Can you work these out from the model? Positions are in its coordinate system, mm. A direction names the side the tool comes from. Round coordinates to 2 decimals unless told otherwise and drop trailing zeros. Write each loop counter-clockwise with the first axis right and the second up, starting at its lowest first coordinate (ties: lowest second). Pieces come first, ordered by that corner, then holes. Notation, with made-up numbers: M 40.5,76.5 L 88.5,76.5 A13 ccw 88.5,83.5 Z; hole C 29.25,40.25 d11. An arc over 180 degrees is marked long. Answer as a JSON object with one key per item and string values. Group by question number.
1) On a 3-axis mill with a long thin cutter (end or side, diameter ignored), from which of +Z, -Z, +X, -X, +Y, -Y can I reach the whole of each face in a straight line? I mean faces 4 (the flat face through (-216.344, -6, 2)), 5 (the flat face through (-97.68, -44, 2)), 6 (the flat face through (-161, -142.256, 2)). Say none if no direction works.
2) Suppose I cut it at A-A, the plane y = -97. Write out the boundary of the cut face in (x, z), and give its area (3 significant figures).
3) Suppose I cut it at B-B, the plane z = 2.7. State how many separate pieces and enclosed holes the cut face has, and give its area (3 significant figures).
4) Suppose I cut it at C-C, the plane y = -68. Write out the boundary of the cut face in (x, z), and give its area (3 significant figures).
5) Please list where these lines run through material, in increasing order: L1, parallel to X at y = -116.5, z = 1.4; L2, parallel to Y at x = -112, z = 1.4; L3, parallel to X at y = -23.5, z = 1.8. Write a range as [from, to].
6) If we mould it in two halves opening along X, with no side actions, what happens to faces 1 (the flat face through (-100.68, -9, 2)), 2 (the flat face through (-116, -1.256, 2)), 3 (the flat face through (-87.68, -73, 2))? For each: +X half, -X half, draft (parallel to the pull), parting line (faces both ways), or undercut.
7) Suppose I cut it at D-D, the plane x = -163. Write out the boundary of the cut face in (y, z).
from build123d import *

# Parameters (mm, degrees)
F0_W     = 3
F0_H     = 5
F1_DEPTH = 4


with BuildPart() as f1:
    # F0 (on Top) → F1 (new body)
    with BuildSketch(Plane.XY):
        with BuildLine():
            Line((-228.3440142274, -137.3912245035), (-231.3440142274, -137.3912245035))
            Line((-231.3440142274, -137.3912245035), (-231.3440142274, -142.256315279))
            Line((-231.3440142274, -142.256315279), (-226.3440142274, -142.256315279))
            Line((-226.3440142274, -142.256315279), (-226.3440142274, -139.3912245035))
            ThreePointArc((-226.3440142274, -139.3912245035), (-227.7582277898, -138.8054380659), (-228.3440142274, -137.3912245035))
        make_face()
        with BuildLine():
            Line((-87.6802765131, -142.256315279), (-87.6802765131, -137.256315279))
            Line((-87.6802765131, -137.256315279), (-90.6802765131, -137.256315279))
            ThreePointArc((-90.6802765131, -137.256315279), (-91.2660629507, -138.6705288414), (-92.6802765131, -139.256315279))
            Line((-92.6802765131, -139.256315279), (-92.6802765131, -142.256315279))
            Line((-92.6802765131, -142.256315279), (-87.6802765131, -142.256315279))
        make_face()
        with BuildLine():
            Line((-87.6802765131, -1.256315279), (-92.6802765131, -1.256315279))
            Line((-92.6802765131, -1.256315279), (-92.6802765131, -4.256315279))
            ThreePointArc((-92.6802765131, -4.256315279), (-91.2660629507, -4.8421017166), (-90.6802765131, -6.256315279))
            Line((-90.6802765131, -6.256315279), (-87.6802765131, -6.256315279))
            Line((-87.6802765131, -6.256315279), (-87.6802765131, -1.256315279))
        make_face()
        with BuildLine():
            Line((-134.6802765131, -1.256315279), (-139.6802765131, -1.256315279))
            Line((-139.6802765131, -1.256315279), (-139.6802765131, -6.256315279))
            Line((-139.6802765131, -6.256315279), (-136.6802765131, -6.256315279))
            ThreePointArc((-136.6802765131, -6.256315279), (-136.0944900755, -4.8421017166), (-134.6802765131, -4.256315279))
            Line((-134.6802765131, -4.256315279), (-134.6802765131, -1.256315279))
        make_face()
        with BuildLine():
            Line((-221.3440142274, -132.256315279), (-231.3440142274, -132.256315279))
            Line((-231.3440142274, -132.256315279), (-231.3440142274, -137.3912245035))
            Line((-231.3440142274, -137.3912245035), (-228.3440142274, -137.3912245035))
            ThreePointArc((-228.3440142274, -137.3912245035), (-226.3440142274, -135.3912245035), (-224.3440142274, -137.3912245035))
            ThreePointArc((-224.3440142274, -137.3912245035), (-224.929800665, -138.8054380659), (-226.3440142274, -139.3912245035))
            Line((-226.3440142274, -139.3912245035), (-226.3440142274, -142.256315279))
            Line((-226.3440142274, -142.256315279), (-221.3440142274, -142.256315279))
            Line((-221.3440142274, -142.256315279), (-221.3440142274, -132.256315279))
        make_face()
        Polygon((-217.9440142274, -132.256315279), (-221.3440142274, -132.256315279), (-221.3440142274, -142.256315279), (-139.3440142274, -142.256315279), (-139.4949736476, -132.256315279), (-142.7440142274, -132.256315279), (-147.4240142274, -132.256315279), (-151.4240142274, -132.256315279), align=None)
        Polygon((-216.3440142274, -11.256315279), (-216.3440142274, -1.256315279), (-221.3440142274, -1.256315279), (-221.3440142274, -6.256315279), (-221.3440142274, -11.256315279), (-217.9440142274, -11.256315279), align=None)
        Polygon((-139.6802765131, -6.256315279), (-139.6802765131, -1.256315279), (-144.6802765131, -1.256315279), (-144.6802765131, -11.256315279), (-142.7440142274, -11.256315279), (-139.6802765131, -11.256315279), align=None)
        Polygon((-134.3440142274, -124.756315279), (-139.3440142274, -124.756315279), (-139.3440142274, -128.856315279), (-139.3440142274, -132.256315279), (-139.4949736476, -132.256315279), (-139.3440142274, -142.256315279), (-129.6802765131, -142.256315279), (-129.6802765131, -124.756315279), align=None)
        with BuildLine():
            Line((-221.3440142274, -6.256315279), (-221.3440142274, -1.256315279))
            Line((-221.3440142274, -1.256315279), (-231.3440142274, -1.256315279))
            Line((-231.3440142274, -1.256315279), (-231.3440142274, -132.256315279))
            Line((-231.3440142274, -132.256315279), (-221.3440142274, -132.256315279))
            Line((-221.3440142274, -132.256315279), (-221.3440142274, -128.856315279))
            Line((-221.3440142274, -128.856315279), (-221.3440142274, -14.656315279))
            Line((-221.3440142274, -14.656315279), (-221.3440142274, -11.256315279))
            Line((-221.3440142274, -11.256315279), (-226.3440142274, -11.256315279))
            Line((-226.3440142274, -11.256315279), (-226.3440142274, -8.256315279))
            ThreePointArc((-226.3440142274, -8.256315279), (-227.7582277898, -4.8421017166), (-224.3440142274, -6.256315279))
            Line((-224.3440142274, -6.256315279), (-221.3440142274, -6.256315279))
        make_face()
        with BuildLine():
            Line((-129.6802765131, -1.256315279), (-134.6802765131, -1.256315279))
            Line((-134.6802765131, -1.256315279), (-134.6802765131, -4.256315279))
            ThreePointArc((-134.6802765131, -4.256315279), (-133.2660629507, -4.8421017166), (-132.6802765131, -6.256315279))
            ThreePointArc((-132.6802765131, -6.256315279), (-134.6802765131, -8.256315279), (-136.6802765131, -6.256315279))
            Line((-136.6802765131, -6.256315279), (-139.6802765131, -6.256315279))
            Line((-139.6802765131, -6.256315279), (-139.6802765131, -11.256315279))
            Line((-139.6802765131, -11.256315279), (-139.4949736476, -11.256315279))
            Line((-139.4949736476, -11.256315279), (-139.3440142274, -11.256315279))
            Line((-139.3440142274, -11.256315279), (-129.6802765131, -11.256315279))
            Line((-129.6802765131, -11.256315279), (-129.6802765131, -6.256315279))
            Line((-129.6802765131, -6.256315279), (-129.6802765131, -1.256315279))
        make_face()
        with BuildLine():
            Line((-92.6802765131, -1.256315279), (-129.6802765131, -1.256315279))
            Line((-129.6802765131, -1.256315279), (-129.6802765131, -6.256315279))
            Line((-129.6802765131, -6.256315279), (-126.6802765131, -6.256315279))
            Line((-126.6802765131, -6.256315279), (-100.6802765131, -6.256315279))
            Line((-100.6802765131, -6.256315279), (-97.6802765131, -6.256315279))
            Line((-97.6802765131, -6.256315279), (-97.6802765131, -11.256315279))
            Line((-97.6802765131, -11.256315279), (-97.6802765131, -14.596315279))
            Line((-97.6802765131, -14.596315279), (-97.6802765131, -74.916315279))
            Line((-97.6802765131, -74.916315279), (-97.6802765131, -78.256315279))
            Line((-97.6802765131, -78.256315279), (-101.0202765131, -78.256315279))
            Line((-101.0202765131, -78.256315279), (-126.3402765131, -78.256315279))
            Line((-126.3402765131, -78.256315279), (-129.6802765131, -78.256315279))
            Line((-129.6802765131, -78.256315279), (-129.6802765131, -108.756315279))
            Line((-129.6802765131, -108.756315279), (-129.6802765131, -111.756315279))
            Line((-129.6802765131, -111.756315279), (-129.6802765131, -114.756315279))
            Line((-129.6802765131, -114.756315279), (-129.6802765131, -124.756315279))
            Line((-129.6802765131, -124.756315279), (-129.6802765131, -142.256315279))
            Line((-129.6802765131, -142.256315279), (-92.6802765131, -142.256315279))
            Line((-92.6802765131, -142.256315279), (-92.6802765131, -139.256315279))
            ThreePointArc((-92.6802765131, -139.256315279), (-94.0944900755, -135.8421017166), (-90.6802765131, -137.256315279))
            Line((-90.6802765131, -137.256315279), (-87.6802765131, -137.256315279))
            Line((-87.6802765131, -137.256315279), (-87.6802765131, -6.256315279))
            Line((-87.6802765131, -6.256315279), (-90.6802765131, -6.256315279))
            ThreePointArc((-90.6802765131, -6.256315279), (-94.0944900755, -7.6705288414), (-92.6802765131, -4.256315279))
            Line((-92.6802765131, -4.256315279), (-92.6802765131, -1.256315279))
        make_face()
        Polygon((-98.1802765131, -124.5755243927), (-124.6802765131, -124.5755243927), (-124.6802765131, -90.2755243927), (-124.6802765131, -88.5755243927), (-122.9802765131, -88.5755243927), (-99.8802765131, -88.5755243927), (-98.1802765131, -88.5755243927), (-98.1802765131, -90.2755243927), align=None, mode=Mode.SUBTRACT)
        Polygon((-129.6802765131, -14.056315279), (-129.6802765131, -11.256315279), (-139.3440142274, -11.256315279), (-139.3440142274, -14.656315279), (-139.3440142274, -114.756315279), (-129.6802765131, -114.756315279), (-129.6802765131, -111.756315279), (-129.6802765131, -108.756315279), (-129.6802765131, -78.256315279), (-129.6802765131, -74.916315279), (-129.6802765131, -27.956315279), (-129.6802765131, -27.456315279), (-129.6802765131, -14.596315279), align=None)
        with BuildLine():
            Line((-139.3440142274, -119.756315279), (-139.3440142274, -124.756315279))
            Line((-139.3440142274, -124.756315279), (-134.3440142274, -124.756315279))
            Line((-134.3440142274, -124.756315279), (-134.3440142274, -121.756315279))
            ThreePointArc((-134.3440142274, -121.756315279), (-135.7582277898, -121.1705288414), (-136.3440142274, -119.756315279))
            Line((-136.3440142274, -119.756315279), (-139.3440142274, -119.756315279))
        make_face()
        with BuildLine():
            Line((-129.6802765131, -114.756315279), (-139.3440142274, -114.756315279))
            Line((-139.3440142274, -114.756315279), (-139.3440142274, -119.756315279))
            Line((-139.3440142274, -119.756315279), (-136.3440142274, -119.756315279))
            ThreePointArc((-136.3440142274, -119.756315279), (-134.3440142274, -117.756315279), (-132.3440142274, -119.756315279))
            ThreePointArc((-132.3440142274, -119.756315279), (-132.929800665, -121.1705288414), (-134.3440142274, -121.756315279))
            Line((-134.3440142274, -121.756315279), (-134.3440142274, -124.756315279))
            Line((-134.3440142274, -124.756315279), (-129.6802765131, -124.756315279))
            Line((-129.6802765131, -124.756315279), (-129.6802765131, -114.756315279))
        make_face()
        with BuildLine():
            Line((-221.3440142274, -11.256315279), (-221.3440142274, -6.256315279))
            Line((-221.3440142274, -6.256315279), (-224.3440142274, -6.256315279))
            ThreePointArc((-224.3440142274, -6.256315279), (-224.929800665, -7.6705288414), (-226.3440142274, -8.256315279))
            Line((-226.3440142274, -8.256315279), (-226.3440142274, -11.256315279))
            Line((-226.3440142274, -11.256315279), (-221.3440142274, -11.256315279))
        make_face()
        Polygon((-126.6802765131, -6.256315279), (-129.6802765131, -6.256315279), (-129.6802765131, -11.256315279), (-126.8802765131, -11.256315279), (-126.6802765131, -11.256315279), align=None)
        with Locations((-99.1802765131, -8.756315279)):
            Rectangle(F0_W, F0_H)
    extrude(amount=F1_DEPTH)


solid = f1.part
Results:
{
 "1": {"face 4": "+Z, -Z, +Y", "face 5": "+Z, -Z", "face 6": "+Z, -Z, +X, -X, -Y"},
 "2": {"outline": "M -231.34,0 L -221.34,0 L -221.34,4 L -231.34,4 Z; M -139.34,0 L -124.68,0 L -124.68,4 L -139.34,4 Z; M -98.18,0 L -87.68,0 L -87.68,4 L -98.18,4 Z", "area": "141 mm^2"},
 "3": {"separate pieces": "1", "enclosed holes": "8", "area": "6,310 mm^2"},
 "4": {"outline": "M -231.34,0 L -221.34,0 L -221.34,4 L -231.34,4 Z; M -139.34,0 L -129.68,0 L -129.68,4 L -139.34,4 Z; M -97.68,0 L -87.68,0 L -87.68,4 L -97.68,4 Z", "area": "119 mm^2"},
 "5": {"L1": "[-231.34, -221.34], [-139.34, -124.68], [-98.18, -87.68]", "L2": "[-142.26, -124.58], [-88.58, -78.26], [-6.26, -1.26]", "L3": "[-231.34, -221.34], [-139.34, -129.68], [-97.68, -87.68]"},
 "6": {"face 1": "undercut", "face 2": "draft", "face 3": "+X half"},
 "7": {"outline": "M -142.26,0 L -132.26,0 L -132.26,4 L -142.26,4 Z"}
}
